Part print with two shaded views. Sizes in mm from the minimum x, y, z corner. A direction names the side the tool comes from. Round coordinates to 2 decimals unless told otherwise and drop trailing zeros. Order: outer loops, then holes, each group sorted by start corner. A loop starts at its lowest first (then second) coordinate and runs counter-clockwise, first axis right, second up. Notation, with made-up numbers: M -17.75,50 L 11.25,50 A19 cw 11.25,63 Z; hole C 81.5,68.25 d6. An arc over 180 degrees is marked long. Return JSON: item names as keys, results as strings. Group by question number.
Item 1: Slice it at D-D on x = 20. Write the cut outline in (y, z).
Item 2: Probe line 1 along X through (y, z) = (71.25, 8); line 2 along Y through (x, z) = (53.5, 10). List the from-to ranges inside material, lowest first.
Item 3: Slice it at A-A on x = 50. Write the cut outline in (y, z), then the cut area to 3 significant figures.
Item 4: Which spindle directions (+Z, -Z, +X, -X, +Y, -Y) get a long thin tool onto all of the face, cutting with end or side? Do the marked faces 1 and 2. Say none if no direction does.
Item 5: Pin check, flat tip, straight feed: pin 1 Ø3 at (x, z) = (50, 8) entering from +Y. Stop position of the tip, or through.
Item 6: Pull direction X, two halves, no side cores. Call the marked faces 3, 4 and 5: pulls with the +X half, pulls with the -X half, needs draft (parallel to the pull), parting line crosses it, or undercut.
Item 7: Slice it at C-C on y = 55. Write the cut outline in (x, z), then the cut area to 3 significant figures.
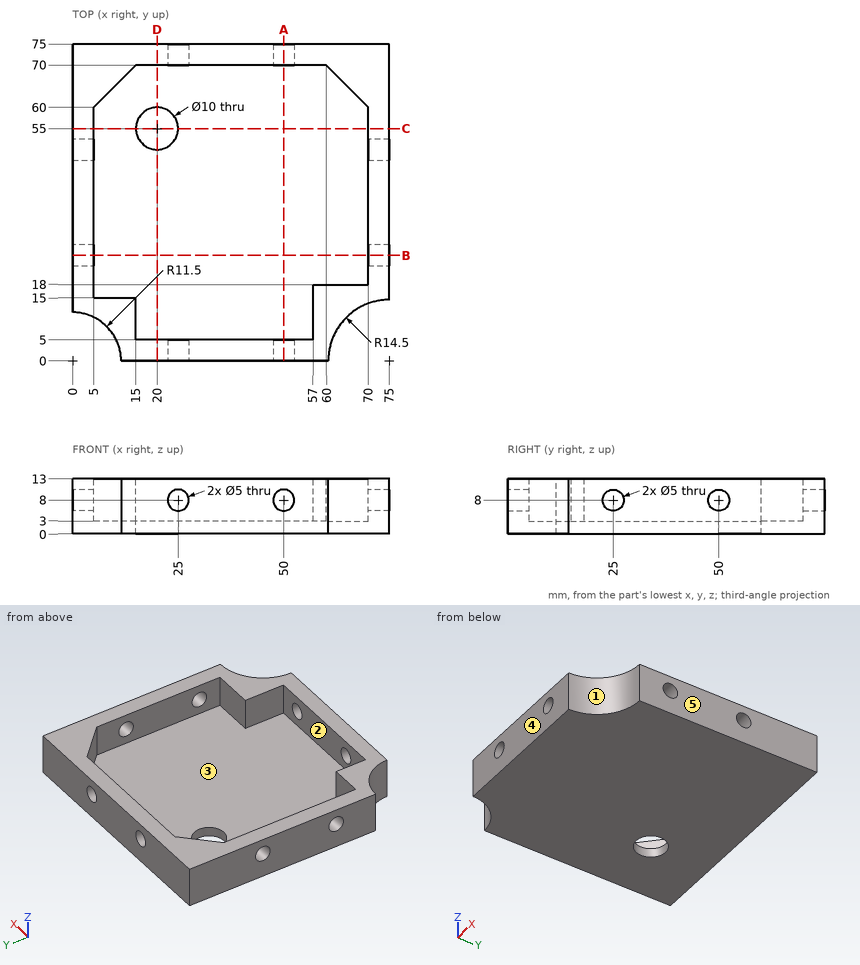
Output values:
{
 "1": {"outline": "M 0,0 L 50,0 L 50,3 L 5,3 L 5,13 L 0,13 Z; M 60,0 L 75,0 L 75,13 L 70,13 L 70,3 L 60,3 Z"},
 "2": {"line 1": "0 to 22.5, 27.5 to 47.5, 52.5 to 75", "line 2": "0 to 5, 70 to 75"},
 "3": {"outline": "M 0,0 L 75,0 L 75,5.5 L 70,5.5 L 70,3 L 5,3 L 5,5.5 L 0,5.5 Z; M 0,10.5 L 5,10.5 L 5,13 L 0,13 Z; M 70,10.5 L 75,10.5 L 75,13 L 70,13 Z", "area": "275 mm²"},
 "4": {"face 1": "+Z, -Z, +X, -Y", "face 2": "+Z"},
 "5": {"pin 1": "through"},
 "6": {"face 3": "undercut", "face 4": "needs draft", "face 5": "pulls with the +X half"},
 "7": {"outline": "M 0,0 L 15,0 L 15,3 L 5,3 L 5,13 L 0,13 Z; M 25,0 L 75,0 L 75,13 L 70,13 L 70,3 L 25,3 Z", "area": "295 mm²"}
}
